Source: three-view drawing plus pictorial views. Frame: mm from the lowest corner of the part. Coordinates: 2 decimals unless noted, no trailing zeros. Write each loop counter-clockwise with the first axis right and the second up, starting at its lowest first coordinate (ties: lowest second). Pieces come first, ordered by that corner, then holes. Notation, with made-up numbers: (30.25, 66.5) -> (69.25, 66.5) arc R25 cw to (69.25, 79.5) -> close; hole circle Ø10 at (-35, -31.5). An arc over 180 degrees is marked (long way). One line per item, written item: value.
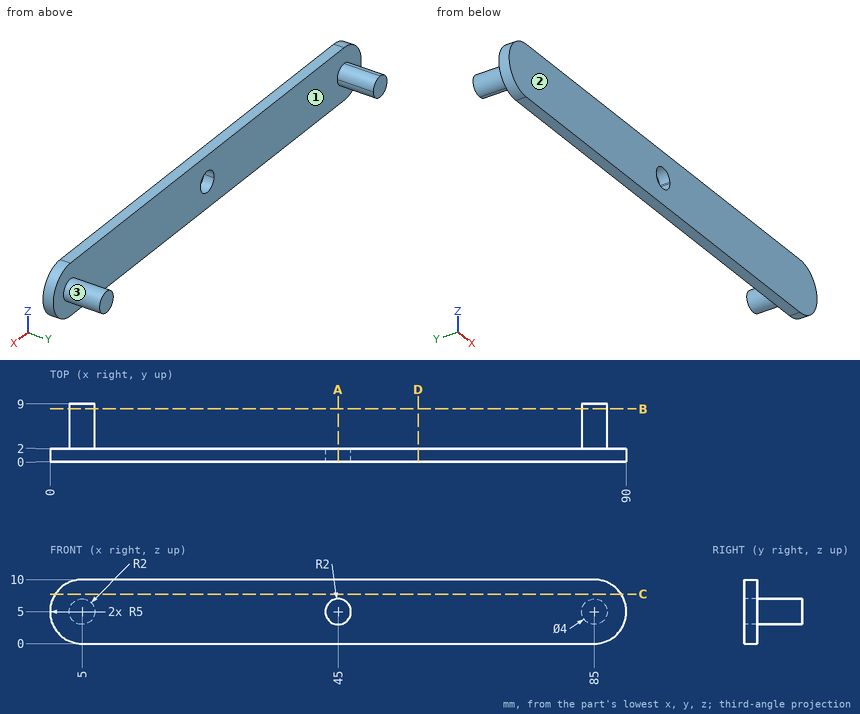
(1) Section A-A (x = 45). Return the cut outline in (y, z).
Responses:
outline: (0, 0) -> (2, 0) -> (2, 3) -> (0, 3) -> close; (0, 7) -> (2, 7) -> (2, 10) -> (0, 10) -> close
(2) Line query: line 1 (Y direction, x = 32, z = 4.75); line 2 (X direction, y = 1.25, z = 5.5); line 3 (X direction, y = 3.25, z = 5.5). Output: solid intervals per line, ascending. Write a range as [from, to].
Responses:
line 1: y = [0, 2]
line 2: x = [0.03, 43.06], [46.94, 89.97]
line 3: x = [3.06, 6.94], [83.06, 86.94]
(3) Section B-B (y = 8.25). Return the cut outline in (x, z), then the cut area to 3 significant figures.
Responses:
outline: circle Ø4 at (5, 5); circle Ø4 at (85, 5)
area: 25.1 mm2
(4) Section D-D (x = 57.5). Return the cut outline in (y, z).
Responses:
outline: (0, 0) -> (2, 0) -> (2, 10) -> (0, 10) -> close
(5) Pull-direction query (X, two-part tool) for the marked faces 1, 2 and 3; classes: released by +X, released by -X, zero draft, split by the parting line, or undercut.
Responses:
face 1: undercut
face 2: zero draft
face 3: undercut
(6) Section C-C (z = 7.75). Return the cut outline in (x, y).
Responses:
outline: (0.82, 0) -> (89.18, 0) -> (89.18, 2) -> (0.82, 2) -> close
(7) First-contact query: pin 1 (2 mm diameter, centred on y = 4.5, z = 4, fed in from +X). Flat tip, straight axial feed; report the tip coordinate or a pass-through.
Responses:
pin 1: stops at x = 87
